CAD build for the part. Positions are in the model's coordinates, mm. A direction names the side the tool comes from. Round coordinates to 2 decimals unless told otherwise and drop trailing zeros. Write each loop counter-clockwise with the first axis right and the second up, starting at its lowest first coordinate (ties: lowest second). Pieces come first, ordered by that corner, then holes. Notation, with made-up numbers: (66, -26) -> (75, -26) arc R20 cw to (75, -22) -> close; hole circle Ø2 at (88, -24.5). An arc over 180 degrees is marked (long way). Put each result on its own line as item: value. Start each with the question number.
1. 3-axis set-ups, long thin cutter, end or side, ignore diameter. For faces 4 (the flat face through (-209.896, 6, -14)), 5 (the cylindrical face through (-211.868, 0.577, 16.062)), 6 (the cylindrical face through (-24.02, -6.15, 75.33)): which of +Z, -Z, +X, -X, +Y, -Y reach the whole face in a straight line?
2. Saw through at A-A on z = 101. List the corners of the cut face in (x, y).
3. Saw through at B-B on x = -66. List the corners of the cut face in (y, z), and give its area (3 significant figures).
4. Pull direction X, two halves, no side cores. Call faces 1 (the flat face through (-86, 4, 145.556)), 2 (the flat face through (-213.896, -1, 17)), 3 (the flat face through (-153, -4.176, -54)): pulls with the +X half, pulls with the -X half, needs draft (parallel to the pull), parting line crosses it, or undercut.
5. Flat gauge pins, fed straight in: P1, Ø4, axis at x = -163.5, z = 20.5, coming from the +Y side; P2, Ø4, axis at x = -36.5, z = 56, coming from the +Y side. Where does each tip first touch, or does it go through?
6. Drill centre lines: line 1 (X direction, y = -1.5, z = -50); line 2 (Z direction, x = -47, y = -0.75); line 3 (X direction, y = 13, z = -82). Where is each one in solid material? Low to high. Write a range as from..to.
from build123d import *

# Parameters (mm, degrees)
SKETCH1_W           = 260
SKETCH1_H           = 260
BOSS_EXTRUDE1_DEPTH = 24
SKETCH2_W           = 252
SKETCH2_H           = 252
CUT_EXTRUDE1_DEPTH  = 16
SKETCH3_W           = 111.5
SKETCH3_H           = 111.5
CUT_EXTRUDE2_DEPTH  = 4
SKETCH4_W           = 111.5
SKETCH4_H           = 111.5
CUT_EXTRUDE3_DEPTH  = 4
SKETCH5_W           = 111.5
SKETCH5_H           = 111.5
CUT_EXTRUDE4_DEPTH  = 4
SKETCH6_W           = 111.5
SKETCH6_H           = 111.5
CUT_EXTRUDE5_DEPTH  = 4
CUT_EXTRUDE6_DEPTH  = 295.911587107
SKETCH8_W           = 20
SKETCH8_H           = 10
CUT_EXTRUDE7_DEPTH  = 334.972898877
CUT_EXTRUDE8_DEPTH  = 260.495566311
CUT_EXTRUDE9_DEPTH  = 260.495566311
CUT_EXTRUDE10_REACH = 339.049
SKETCH11_W          = 20
SKETCH11_H          = 10
SKETCH12_W          = 20
SKETCH12_H          = 10
CUT_EXTRUDE11_DEPTH = 334.972898877
CUT_EXTRUDE12_DEPTH = 260.495566311
SKETCH14_W          = 20
SKETCH14_H          = 10
CUT_EXTRUDE13_DEPTH = 334.972898877
CUT_EXTRUDE14_DEPTH = 260.834464487


with BuildPart() as part:
    # Sketch1 → Boss-Extrude1 (new body)
    with BuildSketch(Plane(origin=(0, 15.823913221, 0), x_dir=(1, 0, 0), z_dir=(0, 1, 0))):
        with Locations((-83.896005, -15.555652519)):
            Rectangle(SKETCH1_W, SKETCH1_H)
    extrude(amount=-BOSS_EXTRUDE1_DEPTH)

    # Sketch2 → Cut-Extrude1 (cut)
    with BuildSketch(Plane(origin=(0, 15.823913221, 0), x_dir=(-1, 0, 0), z_dir=(0, 1, 0))):
        with Locations((83.896005, 15.555652519)):
            Rectangle(SKETCH2_W, SKETCH2_H)
    extrude(amount=-CUT_EXTRUDE1_DEPTH, mode=Mode.SUBTRACT)

    # Sketch3 → Cut-Extrude2 (cut)
    with BuildSketch(Plane(origin=(0, -0.176086779, 0), x_dir=(-1, 0, 0), z_dir=(0, 1, 0))):
        with Locations((13.646005, 85.805652519)):
            Rectangle(SKETCH3_W, SKETCH3_H)
    extrude(amount=-CUT_EXTRUDE2_DEPTH, mode=Mode.SUBTRACT)

    # Sketch4 → Cut-Extrude3 (cut)
    with BuildSketch(Plane(origin=(0, -0.176086779, 0), x_dir=(-1, 0, 0), z_dir=(0, 1, 0))):
        with Locations((154.146005, 85.805652519)):
            Rectangle(SKETCH4_W, SKETCH4_H)
    extrude(amount=-CUT_EXTRUDE3_DEPTH, mode=Mode.SUBTRACT)

    # Sketch5 → Cut-Extrude4 (cut)
    with BuildSketch(Plane(origin=(0, -0.176086779, 0), x_dir=(-1, 0, 0), z_dir=(0, 1, 0))):
        with Locations((154.146005, -54.694347481)):
            Rectangle(SKETCH5_W, SKETCH5_H)
    extrude(amount=-CUT_EXTRUDE4_DEPTH, mode=Mode.SUBTRACT)

    # Sketch6 → Cut-Extrude5 (cut)
    with BuildSketch(Plane(origin=(0, -0.176086779, 0), x_dir=(-1, 0, 0), z_dir=(0, 1, 0))):
        with Locations((13.646005, -54.694347481)):
            Rectangle(SKETCH6_W, SKETCH6_H)
    extrude(amount=-CUT_EXTRUDE5_DEPTH, mode=Mode.SUBTRACT)

    # Sketch7 → Cut-Extrude6 (cut, through all)
    with BuildSketch(Plane(origin=(-209.896005, 0, 0), x_dir=(0, 0, -1), z_dir=(1, 0, 0))):
        with BuildLine():
            Line((15.867865744, 15.823913221), (-46.979170782, 15.823913221))
            ThreePointArc((-46.979170782, 15.823913221), (-15.555652519, 0.573913221), (15.867865744, 15.823913221))
        make_face()
    extrude(amount=-CUT_EXTRUDE6_DEPTH, mode=Mode.SUBTRACT)

    # Sketch8 → Cut-Extrude7 (cut, through all)
    with BuildSketch(Plane(origin=(0, 0, 141.555652519), x_dir=(-1, 0, 0), z_dir=(0, 0, -1))):
        with Locations((168.896005, 7.823913221)):
            Rectangle(SKETCH8_W, SKETCH8_H)
    extrude(amount=-CUT_EXTRUDE7_DEPTH, mode=Mode.SUBTRACT)

    # Sketch9 → Cut-Extrude8 (cut, through all)
    with BuildSketch(Plane(origin=(0, -4.176086779, 0), x_dir=(-1, 0, 0), z_dir=(0, 1, 0))):
        with BuildLine():
            Line((24.071888861, 80.329516126), (19.829248174, 84.572156814))
            ThreePointArc((19.829248174, 84.572156814), (14.879500705, 84.572156814), (14.879500705, 79.622409345))
            Line((14.879500705, 79.622409345), (19.122141392, 75.379768658))
            ThreePointArc((19.122141392, 75.379768658), (24.071888861, 75.379768658), (24.071888861, 80.329516126))
        make_face()
    extrude(amount=-CUT_EXTRUDE8_DEPTH, mode=Mode.SUBTRACT)

    # Sketch10 → Cut-Extrude9 (cut, through all)
    with BuildSketch(Plane(origin=(0, -4.176086779, 0), x_dir=(-1, 0, 0), z_dir=(0, 1, 0))):
        with BuildLine():
            Line((147.962761826, 84.572156814), (143.720121139, 80.329516126))
            ThreePointArc((143.720121139, 80.329516126), (143.720121139, 75.379768658), (148.669868607, 75.379768658))
            Line((148.669868607, 75.379768658), (152.912509294, 79.622409345))
            ThreePointArc((152.912509294, 79.622409345), (152.912509294, 84.572156814), (147.962761826, 84.572156814))
        make_face()
    extrude(amount=-CUT_EXTRUDE9_DEPTH, mode=Mode.SUBTRACT)

    # Sketch11 → Cut-Extrude10 (cut, up to next)
    with BuildSketch(Plane.XY.offset(145.555652519), mode=Mode.PRIVATE) as cut_extrude10_sk1:
        with Locations((1.103995, 7.823913221)):
            Rectangle(SKETCH11_W, SKETCH11_H)
    cut_extrude10_tool1 = extrude(cut_extrude10_sk1.sketch, amount=-CUT_EXTRUDE10_REACH, mode=Mode.PRIVATE) & part.part
    add(cut_extrude10_tool1.solids().sort_by_distance((1.103995, 7.823913, 145.555653))[0], mode=Mode.SUBTRACT)

    # Sketch12 → Cut-Extrude11 (cut, through all)
    with BuildSketch(Plane.XY.offset(-110.444347481)):
        with Locations((-168.896005, 7.823913221)):
            Rectangle(SKETCH12_W, SKETCH12_H)
    extrude(amount=-CUT_EXTRUDE11_DEPTH, mode=Mode.SUBTRACT)

    # Sketch13 → Cut-Extrude12 (cut, through all)
    with BuildSketch(Plane(origin=(0, -4.176086779, 0), x_dir=(-1, 0, 0), z_dir=(0, 1, 0))):
        with BuildLine():
            Line((19.829248174, -53.460851775), (24.071888861, -49.218211088))
            ThreePointArc((24.071888861, -49.218211088), (24.071888861, -44.26846362), (19.122141392, -44.26846362))
            Line((19.122141392, -44.26846362), (14.879500705, -48.511104307))
            ThreePointArc((14.879500705, -48.511104307), (14.879500705, -53.460851775), (19.829248174, -53.460851775))
        make_face()
    extrude(amount=-CUT_EXTRUDE12_DEPTH, mode=Mode.SUBTRACT)

    # Sketch14 → Cut-Extrude13 (cut, through all)
    with BuildSketch(Plane.XY.offset(-110.444347481)):
        with Locations((1.103995, 7.823913221)):
            Rectangle(SKETCH14_W, SKETCH14_H)
    extrude(amount=-CUT_EXTRUDE13_DEPTH, mode=Mode.SUBTRACT)

    # Sketch15 → Cut-Extrude14 (cut, through all)
    with BuildSketch(Plane.XZ.offset(8.176086779)):
        with BuildLine():
            Line((-148.669868607, -44.26846362), (-152.912509294, -48.511104307))
            ThreePointArc((-152.912509294, -48.511104307), (-152.912509294, -53.460851775), (-147.962761826, -53.460851775))
            Line((-147.962761826, -53.460851775), (-143.720121139, -49.218211088))
            ThreePointArc((-143.720121139, -49.218211088), (-143.720121139, -44.26846362), (-148.669868607, -44.26846362))
        make_face()
    extrude(amount=-CUT_EXTRUDE14_DEPTH, mode=Mode.SUBTRACT)


solid = part.part
Return value:
1. face 4: +Y
1. face 5: -X, +Y
1. face 6: +Y, -Y
2. outline: (-213.9, -8.18) -> (46.1, -8.18) -> (46.1, 15.82) -> (42.1, 15.82) -> (42.1, -4.18) -> (-69.4, -4.18) -> (-69.4, -0.18) -> (-98.4, -0.18) -> (-98.4, -4.18) -> (-209.9, -4.18) -> (-209.9, 15.82) -> (-213.9, 15.82) -> close
3. outline: (-8.18, -114.44) -> (15.82, -114.44) -> (15.82, -110.44) -> (-4.18, -110.44) -> (-4.18, 1.06) -> (-0.18, 1.06) -> (-0.18, 30.06) -> (-4.18, 30.06) -> (-4.18, 141.56) -> (15.82, 141.56) -> (15.82, 145.56) -> (-8.18, 145.56) -> close
3. area: 1,320 mm^2
4. face 1: needs draft
4. face 2: pulls with the -X half
4. face 3: undercut
5. P1: stops at y = -0.18
5. P2: stops at y = -4.18
6. line 1: x = -213.9..-209.9, -98.4..-69.4, 42.1..46.1
6. line 2: z = -114.44..-110.44, 1.06..30.06, 141.56..145.56
6. line 3: x = -213.9..-209.9, 42.1..46.1
